Check sheet for the modelled part. Datum: model origin and axes. Units: mm. Face numbers are marked on the shaded views. A direction names the side the tool comes from. Round coordinates to 2 decimals unless told otherwise and drop trailing zeros. Write each loop counter-clockwise with the first axis right and the second up, starting at its lowest first coordinate (ties: lowest second). Pieces come first, ordered by that corner, then holes.
Item 1: Tool access check on the marked faces 1, 2 and 3. Record the directions out of +Z, -Z, +X, -X, +Y, -Y that give a thin tool (end or side, any length) a straight path to the whole face; none if there is none.
Item 2: Go/stop test with flat-tipped pins: pin 1 Ø12 at (x, z) = (-20, 66) entering from +Y; pin 2 Ø4 at (x, y) = (-0.5, -1.5) entering from -Z; pin 3 Ø24 at (x, z) = (0, 0) entering from +Y; pin 4 Ø2 at (y, z) = (-5.5, 45.5) entering from -X. Record where each tip stops, or that it passes through.
Item 3: Release check for a two-part mould opening along Z. For the marked faces 4, 5 and 6 record: +Z half, -Z half, draft (parallel to the pull), parting line (faces both ways), or undercut.
Item 4: Material ranges on line 1 (X direction, y = 10.5, z = 104); line 2 (Z direction, x = 3, y = -10), recorded low to high.
Item 5: Cross-section at B-B on z = 0. Enter the section's corners in (x, y).
Item 6: Cross-section at D-D on z = 96. Enter the section's corners in (x, y).
Item 7: Cross-section at A-A on x = 0. Enter the section's corners in (y, z), plus the area to 3 significant figures.
Item 8: Cross-section at C-C on y = 0. Enter the section's corners in (x, z).
from build123d import *

# Parameters (mm, degrees)
SKETCH1_R                = 30
BOSS_EXTRUDE1_DEPTH      = 17.5
SKETCH2_W                = 33
SKETCH2_H                = 33
BOSS_EXTRUDE2_DEPTH      = 120
SKETCH3_R                = 15
BOSS_EXTRUDE3_DEPTH      = 20
HOLE1_D                  = 30
CUT_EXTRUDE1_DEPTH       = 40
FILLET1_R                = 5
CIRPATTERN1_COUNT        = 4
FILLET1_OF_CIRPATTERN1_R = 5


with BuildPart() as part:
    # Sketch1 → Boss-Extrude1 (new, symmetric)
    with BuildSketch(Plane(origin=(0, 0, 0), x_dir=(1, 0, 0), z_dir=(0, 1, 0))):
        with Locations(Location((0, 0, 0), (0, 0, 270))):
            Circle(SKETCH1_R)
    extrude(amount=BOSS_EXTRUDE1_DEPTH, both=True)

    # Sketch2 → Boss-Extrude2 (add)
    with BuildSketch(Plane.XY):
        Rectangle(SKETCH2_W, SKETCH2_H)
    extrude(amount=BOSS_EXTRUDE2_DEPTH)

    # Sketch3 → Boss-Extrude3 (add)
    with BuildSketch(Plane.XY.offset(120)):
        Circle(SKETCH3_R)
    extrude(amount=BOSS_EXTRUDE3_DEPTH)

    # Hole1 (through all)
    with Locations(Plane(origin=(0, 17.5, 0), x_dir=(1, 0, 0), z_dir=(0, 1, 0))):
        with Locations((0, 0)):
            Hole(HOLE1_D / 2)

    # Sketch6 → Cut-Extrude1 (cut)
    with BuildSketch(Plane.XY.offset(120)):
        with BuildLine():
            Line((11.5, 16.5), (16.5, 16.5))
            Line((16.5, 16.5), (16.5, 11.5))
            ThreePointArc((16.5, 11.5), (12.964466094, 12.964466094), (11.5, 16.5))
        make_face()
    cut_extrude1 = extrude(amount=-CUT_EXTRUDE1_DEPTH, mode=Mode.SUBTRACT)

    # Fillet1
    fillet1_edges = [part.edges().sort_by_distance(p)[0] for p in [
        (12.964466094, 12.964466094, 80),
    ]]
    fillet(fillet1_edges, radius=FILLET1_R - 0.0001)  # a hair under: the kernel refuses the full size

    # CirPattern1: Cut-Extrude1 ×4 about axis
    cirpattern1_axis = Axis((0, 0, 0), (0, 0, 1))
    for i in range(1, CIRPATTERN1_COUNT):
        add(cut_extrude1.rotate(cirpattern1_axis, i * 360 / CIRPATTERN1_COUNT), mode=Mode.SUBTRACT)

    # Fillet1 of CirPattern1
    fillet1_of_cirpattern1_edges = [part.edges().sort_by_distance(p)[0] for p in [
        (-12.964466094, 12.964466094, 80),
        (-12.964466094, -12.964466094, 80),
        (12.964466094, -12.964466094, 80),
    ]]
    fillet(fillet1_of_cirpattern1_edges, radius=FILLET1_OF_CIRPATTERN1_R - 0.0001)  # a hair under: the kernel refuses the full size


solid = part.part
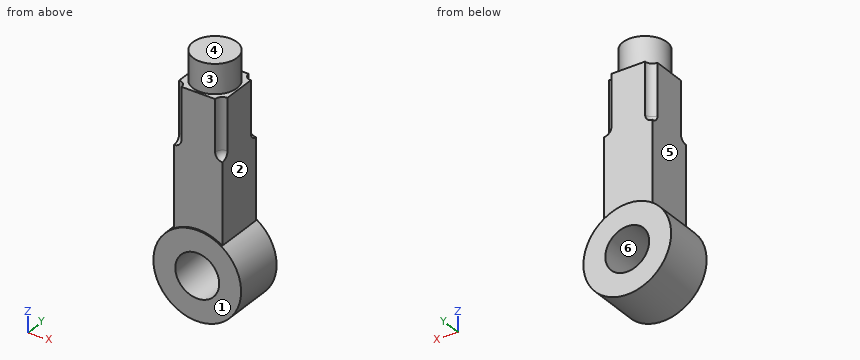
Response values:
1. face 1: +Z, -Z, +X, -X, -Y
1. face 2: +Z, +X, +Y, -Y
1. face 3: +Z
2. pin 1: stops at y = 16.5
2. pin 2: stops at z = -30
2. pin 3: passes through
2. pin 4: stops at x = -16.5
3. face 4: +Z half
3. face 5: draft
3. face 6: undercut
4. line 1: x = -16.5 to 16.5
4. line 2: z = -29.85 to -14.7, 14.7 to 140
5. outline: (-30, -17.5) - (-15, -17.5) - (-15, 17.5) - (-30, 17.5) - close; (15, -17.5) - (30, -17.5) - (30, 17.5) - (15, 17.5) - close
6. outline: (-16.5, -11.5) arc R5 cw to (-11.5, -16.5) - (11.5, -16.5) arc R5 cw to (16.5, -11.5) - (16.5, 11.5) arc R5 cw to (11.5, 16.5) - (-11.5, 16.5) arc R5 cw to (-16.5, 11.5) - close
7. outline: (-17.5, -30) - (17.5, -30) - (17.5, -15) - (-17.5, -15) - close; (-17.5, 15) - (17.5, 15) - (17.5, 30) - (16.5, 30) - (16.5, 120) - (15, 120) - (15, 140) - (-15, 140) - (-15, 120) - (-16.5, 120) - (-16.5, 30) - (-17.5, 30) - close
7. area: 4,620 mm2
8. outline: (-16.5, 25.05) arc R30 ccw (long way) to (16.5, 25.05) - (16.5, 120) - (15, 120) - (15, 140) - (-15, 140) - (-15, 120) - (-16.5, 120) - close; hole circle Ø30 at (0, 0)
